Can you work these out from the model? Positions are in its coordinate system, mm. Face numbers are marked on the shaded views. Round coordinates to 2 decimals unless told otherwise and drop trailing zeros. Loops run counter-clockwise (first coordinate to the right, second up) from the corner with the lowest first, then second, coordinate; pieces in that order, holes last. Notation, with made-up numbers: (-6.75, 31) - (32.25, 31) arc R24 cw to (32.25, 41) - close; hole circle Ø9 at (75, 27). An arc over 180 degrees is marked (long way). Answer as CSV lines item,"result".
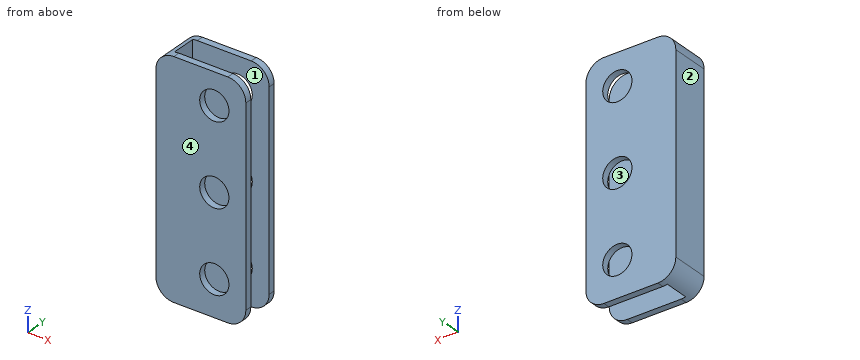
```python
from build123d import *

# Parameters (mm, degrees)
SKETCH1_W           = 20
SKETCH1_H           = 51
BOSS_EXTRUDE1_DEPTH = 1.5
SKETCH2_W           = 3
SKETCH2_H           = 51
BOSS_EXTRUDE2_DEPTH = 5.5
SKETCH3_W           = 20
SKETCH3_H           = 51
BOSS_EXTRUDE3_DEPTH = 1.5
SKETCH4_R           = 3.25
CUT_EXTRUDE1_DEPTH  = 15
FILLET1_R           = 4


with BuildPart() as part:
    # Sketch1 → Boss-Extrude1 (new body)
    with BuildSketch(Plane(origin=(0, 0, 0), x_dir=(1, 0, 0), z_dir=(0, 1, 0))):
        Rectangle(SKETCH1_W, SKETCH1_H)
    extrude(amount=BOSS_EXTRUDE1_DEPTH)

    # Sketch2 → Boss-Extrude2 (add)
    with BuildSketch(Plane(origin=(0, 1.5, 0), x_dir=(1, 0, 0), z_dir=(0, 1, 0))):
        with Locations((-8.5, 0)):
            Rectangle(SKETCH2_W, SKETCH2_H)
    extrude(amount=BOSS_EXTRUDE2_DEPTH)

    # Sketch3 → Boss-Extrude3 (add)
    with BuildSketch(Plane(origin=(0, 7, 0), x_dir=(1, 0, 0), z_dir=(0, 1, 0))):
        Rectangle(SKETCH3_W, SKETCH3_H)
    extrude(amount=BOSS_EXTRUDE3_DEPTH)

    # Sketch4 → Cut-Extrude1 (cut)
    with BuildSketch(Plane(origin=(0, 8.5, 0), x_dir=(1, 0, 0), z_dir=(0, 1, 0))):
        with Locations(Location((3, 17.5, 0), (0, 0, 270))):
            Circle(SKETCH4_R)
        with Locations(Location((3, -0.5, 0), (0, 0, 270))):
            Circle(SKETCH4_R)
        with Locations(Location((3, -18.5, 0), (0, 0, 270))):
            Circle(SKETCH4_R)
    extrude(amount=-CUT_EXTRUDE1_DEPTH, mode=Mode.SUBTRACT)

    # Fillet1
    # the kernel refuses this fillet: 4 mm, written as the material it takes off along each edge
    with BuildSketch(Plane(origin=(-10, 18.5, 25.5), x_dir=(1, 0, 0), z_dir=(0, -1, 0)), Plane(origin=(-10, 18.5, -25.5), x_dir=(0, 0, 1), z_dir=(0, -1, 0))) as fillet1_piece_1:
        with BuildLine():
            CenterArc((FILLET1_R, -FILLET1_R), FILLET1_R, 90, 90)
            Line((0, -FILLET1_R), (0, 0))
            Line((0, 0), (FILLET1_R, 0))
        make_face()
    extrude(amount=28.5, mode=Mode.SUBTRACT)
    with BuildSketch(Plane(origin=(10, -10, 25.5), x_dir=(-1, 0, 0), z_dir=(0, 1, 0)), Plane(origin=(10, -3, 25.5), x_dir=(-1, 0, 0), z_dir=(0, 1, 0)), Plane(origin=(10, -10, -25.5), x_dir=(0, 0, 1), z_dir=(0, 1, 0)), Plane(origin=(10, -3, -25.5), x_dir=(0, 0, 1), z_dir=(0, 1, 0))) as fillet1_piece_2:
        with BuildLine():
            CenterArc((FILLET1_R, -FILLET1_R), FILLET1_R, 90, 90)
            Line((0, -FILLET1_R), (0, 0))
            Line((0, 0), (FILLET1_R, 0))
        make_face()
    extrude(amount=21.5, mode=Mode.SUBTRACT)


solid = part.part
```
Q1. I'm going to push a flat-ended pin straight in: pin 1 Ø6 at (x, z) = (3, 0.5) entering from +Y. Where does the tip first touch, or does it pass through?
Checks:
pin 1,"through"
Q2. We'd pull the mould along Y, two halves only. Please class the marked faces 1, 2, 3 and 4: pulls with the +Y half, pulls with the -Y half, needs draft (parallel to the pull), parting line crosses it, or undercut.
Checks:
face 1,"undercut"
face 2,"needs draft"
face 3,"undercut"
face 4,"pulls with the -Y half"
Q3. Imagine slicing it at C-C (z = -5.5). Write out the boundary of the cut face in (x, y), then the cut area to 3 significant figures.
Checks:
outline,"(-10, 0) - (10, 0) - (10, 1.5) - (-7, 1.5) - (-7, 7) - (10, 7) - (10, 8.5) - (-10, 8.5) - close"
area,"76.5 mm²"
Q4. Imagine slicing it at D-D (x = 6.75). Write out the boundary of the cut face in (y, z).
Checks:
outline,"(0, -25.43) - (1.5, -25.43) - (1.5, 25.43) - (0, 25.43) - close; (7, -25.43) - (8.5, -25.43) - (8.5, 25.43) - (7, 25.43) - close"
Q5. Imagine slicing it at B-B (x = 3). Count the separate pieces of the cut face and the enclosed holes in it, then the cut area to 3 significant figures.
Checks:
separate pieces,"8"
enclosed holes,"0"
area,"94.5 mm²"
Q6. Imagine slicing it at A-A (z = 18.5). Write out the boundary of the cut face in (x, y), then the cut area to 3 significant figures.
Checks:
outline,"(-10, 0) - (-0.25, 0) - (-0.25, 1.5) - (-7, 1.5) - (-7, 7) - (-0.25, 7) - (-0.25, 8.5) - (-10, 8.5) - close; (6.25, 0) - (10, 0) - (10, 1.5) - (6.25, 1.5) - close; (6.25, 7) - (10, 7) - (10, 8.5) - (6.25, 8.5) - close"
area,"57.0 mm²"
Q7. If I drill on line 1 along Y through (x, z) = (3.5, -9); line 2 along Z through (x, y) = (3.75, 1); line 3 along X through (y, z) = (7.95, 18.5), over which ranges is the centre line in solid material (lowest first)? Write a range as [from, to].
Checks:
line 1,"[0, 1.5], [7, 8.5]"
line 2,"[-25.5, -20.66], [-14.34, -2.66], [3.66, 15.34], [21.66, 25.5]"
line 3,"[-10, -0.25], [6.25, 10]"
